Source: CAD feature listing. Evaluate the final solid. Frame: model axes, mm. Face numbers are marked on the shaded views. A direction names the side the tool comes from. Round coordinates to 2 decimals unless told otherwise and drop trailing zeros. Write each loop counter-clockwise with the first axis right and the second up, starting at its lowest first coordinate (ties: lowest second). Pieces come first, ordered by that corner, then holes.
from build123d import *

# Parameters (mm, degrees)
SKETCH1_W                 = 50
SKETCH1_H                 = 25
BOSS_EXTRUDE1_DEPTH       = 3.175
M4X0_7_TAPPED_HOLE1_D     = 3.3
M4X0_7_TAPPED_HOLE1_DEPTH = 10.1
M4X0_7_TAPPED_HOLE1_TIP   = 0.991420021
BOSS_EXTRUDE2_START       = -7.5
BOSS_EXTRUDE2_DEPTH       = 10


with BuildPart() as part:
    # Sketch1 → Boss-Extrude1 (new body)
    with BuildSketch(Plane(origin=(0, 0, 0), x_dir=(1, 0, 0), z_dir=(0, 1, 0))):
        with Locations((25, 12.5)):
            Rectangle(SKETCH1_W, SKETCH1_H)
    extrude(amount=BOSS_EXTRUDE1_DEPTH)

    # M4x0.7 Tapped Hole1
    with Locations(Plane(origin=(5, 3.175, -21.5), x_dir=(0, 0, 1), z_dir=(0, 1, 0))):
        with Locations((0, 0), (0, 40), (18, 0), (18, 40)):
            Hole(M4X0_7_TAPPED_HOLE1_D / 2, depth=M4X0_7_TAPPED_HOLE1_DEPTH)
            with Locations((0, 0, -(M4X0_7_TAPPED_HOLE1_DEPTH + M4X0_7_TAPPED_HOLE1_TIP / 2))):  # 118° drill point
                Cone(0, M4X0_7_TAPPED_HOLE1_D / 2, M4X0_7_TAPPED_HOLE1_TIP, mode=Mode.SUBTRACT)

    # Sketch4 → Boss-Extrude2 (add)
    with BuildSketch(Plane.XY.offset(BOSS_EXTRUDE2_START)):
        Polygon((0, 3.175), (5, 3.175), (2.5, 6.35), align=None)
        Polygon((5, 3.175), (10, 3.175), (7.5, 6.35), align=None)
        Polygon((10, 3.175), (15, 3.175), (12.5, 6.35), align=None)
        Polygon((15, 3.175), (20, 3.175), (17.5, 6.35), align=None)
        Polygon((20, 3.175), (25, 3.175), (22.5, 6.35), align=None)
        Polygon((27.5, 6.35), (25, 3.175), (30, 3.175), align=None)
        Polygon((32.5, 6.35), (30, 3.175), (35, 3.175), align=None)
        Polygon((37.5, 6.35), (35, 3.175), (40, 3.175), align=None)
        Polygon((42.5, 6.35), (40, 3.175), (45, 3.175), align=None)
        Polygon((47.5, 6.35), (45, 3.175), (50, 3.175), align=None)
    extrude(amount=-BOSS_EXTRUDE2_DEPTH)


solid = part.part
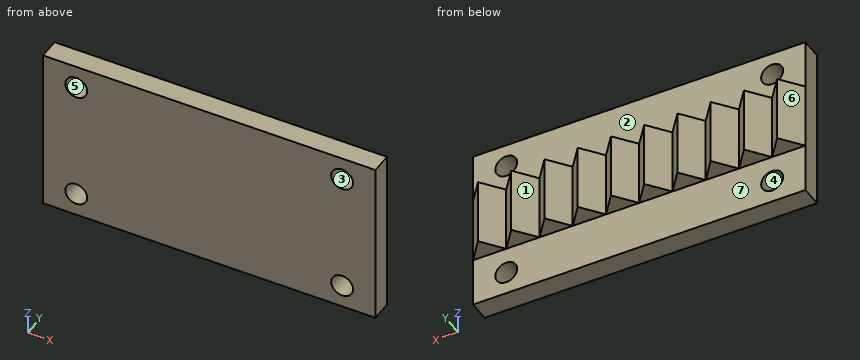
1) Material intervals for line 1 (X direction, y = 1.4, z = -3.5); line 2 (X direction, y = 2.75, z = -22.25); line 3 (Y direction, x = 33, z = -5.75) (3 decimals), sorted ascending.
Taken from the geometry:
line 1: x = 0 to 3.35, 6.65 to 43.35, 46.65 to 50
line 2: x = 0 to 3.53, 6.47 to 43.53, 46.47 to 50
line 3: y = 0 to 3.175
2) Reachability of the marked faces 1, 2 and 3 from +Z, -Z, +X, -X, +Y, -Y: full face, straight path, thin tool, end or side. Return the list, or none.
Taken from the geometry:
face 1: +Z, -Z, +Y
face 2: +Z, +X, -X, +Y
face 3: +Y, -Y
3) Section query C-C on y = 1.75. Return the cut outline in (x, z).
Taken from the geometry:
outline: (0, -25) - (50, -25) - (50, 0) - (0, 0) - close; hole circle Ø3.3 at (5, -21.5); hole circle Ø3.3 at (5, -3.5); hole circle Ø3.3 at (45, -21.5); hole circle Ø3.3 at (45, -3.5)
4) Section query A-A on z = -3.5. Return the cut outline in (x, y) (3 decimals).
Taken from the geometry:
outline: (0, 0) - (3.35, 0) - (3.35, 3.175) - (0, 3.175) - close; (6.65, 0) - (43.35, 0) - (43.35, 3.175) - (6.65, 3.175) - close; (46.65, 0) - (50, 0) - (50, 3.175) - (46.65, 3.175) - close
5) Pull-direction query (X, two-part tool) for the marked faces 4, 5, 6 and 7; classes: released by +X, released by -X, zero draft, split by the parting line, or undercut.
Taken from the geometry:
face 4: undercut
face 5: undercut
face 6: released by -X
face 7: zero draft
6) Section query D-D on z = -14.5. Return the cut outline in (x, y) (3 decimals).
Taken from the geometry:
outline: (0, 0) - (50, 0) - (50, 3.175) - (47.5, 6.35) - (45, 3.175) - (42.5, 6.35) - (40, 3.175) - (37.5, 6.35) - (35, 3.175) - (32.5, 6.35) - (30, 3.175) - (27.5, 6.35) - (25, 3.175) - (22.5, 6.35) - (20, 3.175) - (17.5, 6.35) - (15, 3.175) - (12.5, 6.35) - (10, 3.175) - (7.5, 6.35) - (5, 3.175) - (2.5, 6.35) - (0, 3.175) - close
7) Contact query for flat-ended pins moving along their axis: P1, Ø1.6, axis at x = 43.5, y = 4.5, coming from the +Z side; P2, Ø2.5, axis at x = 26.5, y = 4.5, coming from the -Z side; P3, Ø5.5, axis at x = 45, z = -3.5, coming from the +Y side (3 decimals). Output: stop coordinate, or through.
Taken from the geometry:
P1: stops at z = -7.5
P2: stops at z = -17.5
P3: stops at y = 3.175
8) Section query B-B on x = 31.5. Return the cut outline in (y, z) (3 decimals), then the cut area to 3 significant figures.
Taken from the geometry:
outline: (0, -25) - (3.175, -25) - (3.175, -17.5) - (5.08, -17.5) - (5.08, -7.5) - (3.175, -7.5) - (3.175, 0) - (0, 0) - close
area: 98.4 mm2
